Work out the finished part from the listing and answer in its coordinate system (mm). Give positions to 0.01 mm unless a question says otherwise; leave off trailing zeros. Write each loop counter-clockwise with the first axis right and the second up, starting at its lowest first coordinate (ties: lowest second). Pieces come first, ordered by that corner, then holes. Notation, with made-up numbers: (14.5, 74) - (53.5, 74) arc R34 ccw to (53.5, 106) - close; hole circle Ø11 at (-28, -15). An arc over 180 degrees is marked (long way). Write each question's results on one line, items separated by ' | '. Start each with the question number.
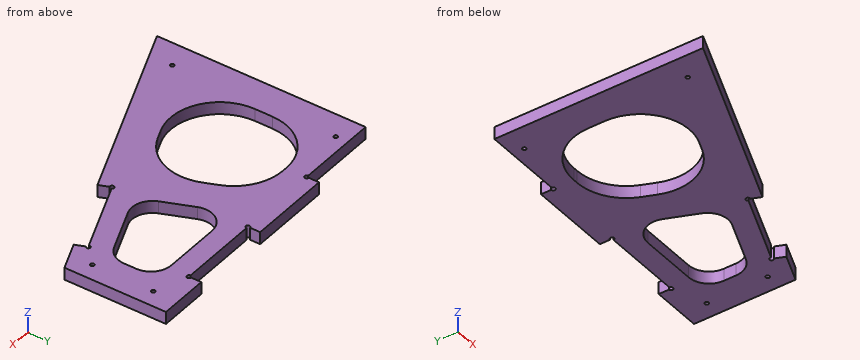
from build123d import *

# Parameters (mm, degrees)
BOSS_EXTRUDE1_DEPTH              = 19.05
CUT_EXTRUDE2_DEPTH               = 7658.473916494
FILLET1_R                        = 76.2
FILLET2_R                        = 31.75
SKETCH2_W                        = 127
SKETCH2_H                        = 19.05
CUT_EXTRUDE1_DEPTH               = 7658.473916494
F_1_4_0_25_DIAMETER_HOLE1_D      = 6.35
F_15_64_0_23438_DIAMETER_HOLE1_D = 5.953252


with BuildPart() as part:
    # Sketch1 → Boss-Extrude1 (new body)
    with BuildSketch(Plane.XY):
        Polygon((3140.71, 6983.72999014), (2683.51, 6983.72999014), (2683.51, 6641.741886848), (3140.71, 6826.4626773), align=None)
    extrude(amount=BOSS_EXTRUDE1_DEPTH)

    # Sketch6 → Cut-Extrude2 (cut, through all)
    with BuildSketch(Plane(origin=(0, 0, 0), x_dir=(-1, 0, 0), z_dir=(0, 0, -1))):
        Polygon((-2923.76447292, 6932.92999014), (-3089.91, 6932.92999014), (-3089.91, 6860.727709955), (-2972.15765047, 6813.152672592), align=None)
        Polygon((-2925.056710658, 6794.122657646), (-2734.31, 6717.055984048), (-2734.31, 6932.92999014), (-2868.974907992, 6932.92999014), align=None)
    extrude(amount=-CUT_EXTRUDE2_DEPTH, mode=Mode.SUBTRACT)

    # Fillet1
    fillet1_edges = [part.edges().sort_by_distance(p)[0] for p in [
        (2925.056710658, 6794.122657646, 9.525),
        (2868.974907992, 6932.92999014, 9.525),
        (2734.31, 6932.92999014, 9.525),
        (2734.31, 6717.055984048, 9.525),
    ]]
    fillet(fillet1_edges, radius=FILLET1_R)

    # Fillet2
    fillet2_edges = [part.edges().sort_by_distance(p)[0] for p in [
        (2972.15765047, 6813.152672592, 9.525),
        (3089.91, 6860.727709955, 9.525),
        (3089.91, 6932.92999014, 9.525),
        (2923.76447292, 6932.92999014, 9.525),
    ]]
    fillet(fillet2_edges, radius=FILLET2_R)

    # Sketch2 → Cut-Extrude1 (cut, through all)
    with BuildSketch(Plane(origin=(0, 0, 0), x_dir=(-1, 0, 0), z_dir=(0, 0, -1))):
        with Locations((-2747.01, 6974.20499014)):
            Rectangle(SKETCH2_W, SKETCH2_H)
        with Locations((-3001.01, 6974.20499014)):
            Rectangle(SKETCH2_W, SKETCH2_H)
        Polygon((-2977.551881268, 6760.542518374), (-3095.304230798, 6808.117555738), (-3088.167975193, 6825.780408168), (-2970.415625663, 6778.205370804), align=None)
    extrude(amount=-CUT_EXTRUDE1_DEPTH, mode=Mode.SUBTRACT)

    # 1/4 (0.25) Diameter Hole1 (through all)
    with Locations(Plane(origin=(0, 0, 0), x_dir=(-1, 0, 0), z_dir=(0, 0, -1))):
        with Locations((-3088.167975193, 6825.780408168), (-2970.415625663, 6778.205370804), (-2937.51, 6964.67999014), (-3064.51, 6964.67999014), (-2810.51, 6964.67999014)):
            Hole(F_1_4_0_25_DIAMETER_HOLE1_D / 2)

    # 15/64 (0.23438) Diameter Hole1 (through all)
    with Locations(Plane.YX):
        with Locations((6692.541891629, 2721.610000001), (6945.629994921, 2721.610000001), (6945.629994921, 3115.310000001), (6851.60701674, 3115.310000001)):
            Hole(F_15_64_0_23438_DIAMETER_HOLE1_D / 2)


solid = part.part
Q1. A cutting plane is placed at A-A, the plane y = 6926. Write down the section's boundary in (x, z).
Q2. Given pin 1 (8 mm diameter, centred on x = 2815.5, z = 10.5, fed in from -Y); pin 2 (9.5 mm diameter, centred on x = 2757, z = 11.5, fed in from +Y), each flat-ended and moving along its own axis, determine where each tip first touches the part or whether it passes through.
Q3. A cutting plane is placed at D-D, the plane y = 6682. Write down the section's boundary in (x, z), and give its area (3 significant figures).
Q4. A cutting plane is placed at C-C, the plane x = 3105. Write down the section's boundary in (y, z), and give its area (3 significant figures).
Q5. Consider L1, parallel to X at y = 6918.5, z = 14.75; L2, parallel to X at y = 6944, z = 15.5; L3, parallel to X at y = 6849.5, z = 15. Determine where each line is inside the solid, lowest interval first.
Q6. A cutting plane is placed at B-B, the plane z = 5.5. Give the number of separate pieces and of enclosed holes in the cut face, and give its area (3 significant figures).
Result:
1) outline: (2683.51, 0) - (2778.76, 0) - (2778.76, 19.05) - (2683.51, 19.05) - close; (2849.33, 0) - (2951.04, 0) - (2951.04, 19.05) - (2849.33, 19.05) - close; (3077.96, 0) - (3140.71, 0) - (3140.71, 19.05) - (3077.96, 19.05) - close
2) pin 1: stops at y = 6693.45 | pin 2: stops at y = 6964.68
3) outline: (2683.51, 0) - (2783.15, 0) - (2783.15, 19.05) - (2683.51, 19.05) - close | area: 1,900 mm2
4) outline: (6812.03, 0) - (6983.73, 0) - (6983.73, 19.05) - (6812.03, 19.05) - close | area: 3,270 mm2
5) L1: x = 2683.51 to 2765.89, 2862.2 to 2944.23, 3084.77 to 3140.71 | L2: x = 2683.51 to 2719.12, 2724.1 to 3112.82, 3117.8 to 3140.71 | L3: x = 2683.51 to 2734.31, 2900.9 to 2957.47, 3062.12 to 3113.21, 3117.41 to 3140.71
6) separate pieces: 1 | enclosed holes: 6 | area: 69,400 mm2
